Autodesk Inventor part; units mm, degrees
ref_plane "YZ Plane" through (0, 0, 0) normal (1, 0, 0) x (0, 1, 0)
ref_plane "XZ Plane" through (0, 0, 0) normal (0, 1, 0) x (-1, 0, 0)
ref_plane "XY Plane" through (0, 0, 0) normal (0, 0, 1) x (1, 0, 0)
sketch "Sketch1" plane through (0, 0, 0) normal (0, 1, 0) x (-1, 0, 0)
  circle A0 centre (0, 0) radius 200
  dimension "d0" = 400
ref_plane "Work Plane1" through (0, 3, 0) normal (0, 1, 0) x (1, 0, 0)
sketch "Sketch2" plane through (0, 3, 0) normal (0, 1, 0) x (1, 0, 0)
  line L0 (-63.5, -143.5) -> (63.5, -143.5)
  line L1 (63.5, -143.5) -> (63.5, 143.5)
  line L2 (63.5, 143.5) -> (-63.5, 143.5)
  line L3 (-63.5, 143.5) -> (-63.5, -143.5)
  line L4 (-63.5, -143.5) -> (63.5, 143.5) construction
  line L5 (63.5, -143.5) -> (-63.5, 143.5) construction
  point P0 (0, 0)
  dimension "d3" = 127
  dimension "d4" = 287
extrude "Extrusion2" [suppressed]
ref_plane "Work Plane4" through (0, 3, 0) normal (0, 1, 0) x (1, 0, 0)
sketch "Sketch3" plane through (0, 3, 0) normal (0, 1, 0) x (1, 0, 0)
  line L0 (-63.5, 143.5) -> (-63.5, -143.5)
  line L1 (-63.5, 0) -> (-123.5, 0)
  line L2 (-123.5, 0) -> (-93.5, 0)
  line L3 (-93.5, 0) -> (-119.5, 0)
  circle A0 centre (-119.5, 0) radius 2.5
  circle A1 centre (-117.932, -8.8925) radius 2.5
  circle A2 centre (-113.4172, -16.7125) radius 2.5
  circle A3 centre (-106.5, -22.5167) radius 2.5
  circle A4 centre (-98.0149, -25.605) radius 2.5
  circle A5 centre (-88.9851, -25.605) radius 2.5
  circle A6 centre (-80.5, -22.5167) radius 2.5
  circle A7 centre (-73.5828, -16.7125) radius 2.5
  circle A8 centre (-69.068, -8.8925) radius 2.5
  circle A9 centre (-67.5, 0) radius 2.5
  circle A10 centre (-69.068, 8.8925) radius 2.5
  circle A11 centre (-73.5828, 16.7125) radius 2.5
  circle A12 centre (-80.5, 22.5167) radius 2.5
  circle A13 centre (-88.9851, 25.605) radius 2.5
  circle A14 centre (-98.0149, 25.605) radius 2.5
  circle A15 centre (-106.5, 22.5167) radius 2.5
  circle A16 centre (-113.4172, 16.7125) radius 2.5
  circle A17 centre (-117.932, 8.8925) radius 2.5
  line L4 (-93.5, 0) -> (-110.5, 0)
  line L5 (-110.5, 0) -> (-92.5712, 0)
  line L6 (-93.5, 0) -> (-103.5, 0)
  circle A18 centre (-110.5, 0) radius 2
  circle A19 centre (-103.5, 0) radius 1.5
  circle A20 centre (-109.4748, -5.8143) radius 2
  circle A21 centre (-106.5228, -10.9274) radius 2
  circle A22 centre (-102, -14.7224) radius 2
  circle A23 centre (-96.452, -16.7417) radius 2
  circle A24 centre (-90.548, -16.7417) radius 2
  circle A25 centre (-85, -14.7224) radius 2
  circle A26 centre (-80.4772, -10.9274) radius 2
  circle A27 centre (-77.5252, -5.8143) radius 2
  circle A28 centre (-76.5, 0) radius 2
  circle A29 centre (-77.5252, 5.8143) radius 2
  circle A30 centre (-80.4772, 10.9274) radius 2
  circle A31 centre (-85, 14.7224) radius 2
  circle A32 centre (-90.548, 16.7417) radius 2
  circle A33 centre (-96.452, 16.7417) radius 2
  circle A34 centre (-102, 14.7224) radius 2
  circle A35 centre (-106.5228, 10.9274) radius 2
  circle A36 centre (-109.4748, 5.8143) radius 2
  circle A37 centre (-101.5902, -5.8779) radius 1.5
  circle A38 centre (-96.5902, -9.5106) radius 1.5
  circle A39 centre (-90.4098, -9.5106) radius 1.5
  circle A40 centre (-85.4098, -5.8779) radius 1.5
  circle A41 centre (-83.5, 0) radius 1.5
  circle A42 centre (-85.4098, 5.8779) radius 1.5
  circle A43 centre (-90.4098, 9.5106) radius 1.5
  circle A44 centre (-96.5902, 9.5106) radius 1.5
  circle A45 centre (-101.5902, 5.8779) radius 1.5
  point P0 (0, 0)
  dimension "d7" = 60
  dimension "d8" = 30
  dimension "d9" = 26
  dimension "d10" = 5
  dimension "d13" = 360
  dimension "d15" = 17
  dimension "d16" = 10
  dimension "d18" = 4
  dimension "d19" = 3
  dimension "d22" = 360
  dimension "d26" = 360
extrude "Extrusion3" [suppressed]
ref_plane "Work Plane2" through (0, 3, 0) normal (0, 1, 0) x (1, 0, 0)
sketch "Sketch4" plane through (0, 3, 0) normal (0, 1, 0) x (1, 0, 0)
  line L0 (0, 0) -> (0, -170)
  line L1 (0, -170) -> (0, 170)
  line L2 (0, -170) -> (-40, -170)
  line L3 (-40, -170) -> (-65, -170)
  line L4 (-65, -170) -> (0, -170)
  line L5 (0, -170) -> (65, -170)
  line L6 (0, 170) -> (-65, 170)
  line L7 (-65, 170) -> (0, 170)
  line L8 (0, 170) -> (65, 170)
  circle A0 centre (65, 170) radius 1.5
  circle A1 centre (-65, 170) radius 1.5
  circle A2 centre (-65, -170) radius 1.5
  circle A3 centre (65, -170) radius 1.5
  dimension "d30" = 170
  dimension "d31" = 340
  dimension "d32" = 40
  dimension "d33" = 25
  dimension "d34" = 65
  dimension "d35" = 65
  dimension "d36" = 65
  dimension "d37" = 65
  dimension "d38" = 65
  dimension "d39" = 3
  dimension "d40" = 3
  dimension "d41" = 3
  dimension "d42" = 3
extrude "Extrusion4" [suppressed]
ref_plane "Work Plane3" through (0, 3, 0) normal (0, 1, 0) x (1, 0, 0)
sketch "Sketch5" plane through (0, 3, 0) normal (0, 1, 0) x (1, 0, 0)
  circle A0 centre (0, 0) radius 201
  circle A1 centre (0, 0) radius 200
  dimension "d45" = 402
  dimension "d46" = 400
extrude "Extrusion5" add sketch "Sketch5" along normal blind 100 and the other way blind 3
sketch "Sketch6" plane through (0, 0, 0) normal (1, 0, 0) x (0, 1, 0)
  line L0 (0, -200) -> (0, 200)
  line L1 (0, -200) -> (0, 200)
  line L2 (0, 200) -> (103, 201)
  line L3 (0, 201) -> (103, 201)
  line L4 (103, -201) -> (103, 201)
  line L5 (103, -201) -> (103, 201)
  line L6 (103, 201) -> (103, 0)
  line L7 (73, -100) -> (133, -100)
  line L8 (133, -100) -> (133, 100)
  line L9 (133, 100) -> (73, 100)
  line L10 (73, 100) -> (73, -100)
  line L11 (73, -100) -> (133, 100) construction
  line L12 (133, -100) -> (73, 100) construction
  point P0 (0, 0)
  dimension "d51" = 60
  dimension "d52" = 200
extrude "Extrusion6" cut sketch "Sketch6" along normal blind 300
properties part number "border" material "PC/ABS Plastic"
Input: part model. Units: mm. Frame: model coordinates. Give positions to 0.01 mm unless a question says otherwise; leave off trailing zeros. Loops run counter-clockwise (first coordinate to the right, second up) from the corner with the lowest first, then second, coordinate; pieces in that order, holes last.
1) Section query A-A on x = 0. Return the cut outline in (y, z).
A:
outline: (0, -201) - (103, -201) - (103, -200) - (0, -200) - close; (0, 200) - (103, 200) - (103, 201) - (0, 201) - close
2) Line query: L1, parallel to Z at x = 0, y = 46.5; L2, parallel to Z at x = 74, y = 92. Output: solid intervals per line, ascending.
A:
L1: z = -201 to -200, 200 to 201
L2: z = -186.88 to -185.81, 185.81 to 186.88
3) Section query C-C on y = 60.5. Return the cut outline in (x, z), and give its area (3 significant figures).
A:
outline: circle Ø402 at (0, 0); hole circle Ø400 at (0, 0)
area: 1,260 mm2
4) Contact query for flat-ended pins moving along their axis: pin 1 (5 mm diameter, centred on y = 66, z = 83, fed in from -X); pin 2 (1.5 mm diameter, centred on y = 74.5, z = -27.5, fed in from +X); pin 3 (4 mm diameter, centred on y = 25.5, z = 38.5, fed in from -X). Output: stop coordinate, or through.
A:
pin 1: stops at x = -184.18
pin 2: stops at x = -197.99
pin 3: stops at x = -197.66
5) Section query B-B on z = 0. Return the cut outline in (x, y), and give its area (3 significant figures).
A:
outline: (-201, 0) - (-200, 0) - (-200, 103) - (-201, 103) - close; (200, 0) - (201, 0) - (201, 73) - (200, 73) - close
area: 176 mm2
6) Mould query, pull axis Z, two halves, no side actions, for faces 1 (the cylindrical face through (-199.807, 52.221, -8.794)), 2 (the cylindrical face through (-200.806, 52.221, -8.838)). Classes: released by +Z, released by -Z, zero draft, split by the parting line, or undercut.
A:
face 1: undercut
face 2: split by the parting line
7) Section query D-D on y = 86. Return the cut outline in (x, z).
A:
outline: (173.21, -100) arc R200 cw (long way) to (173.21, 100) - (174.36, 100) arc R201 ccw (long way) to (174.36, -100) - close
